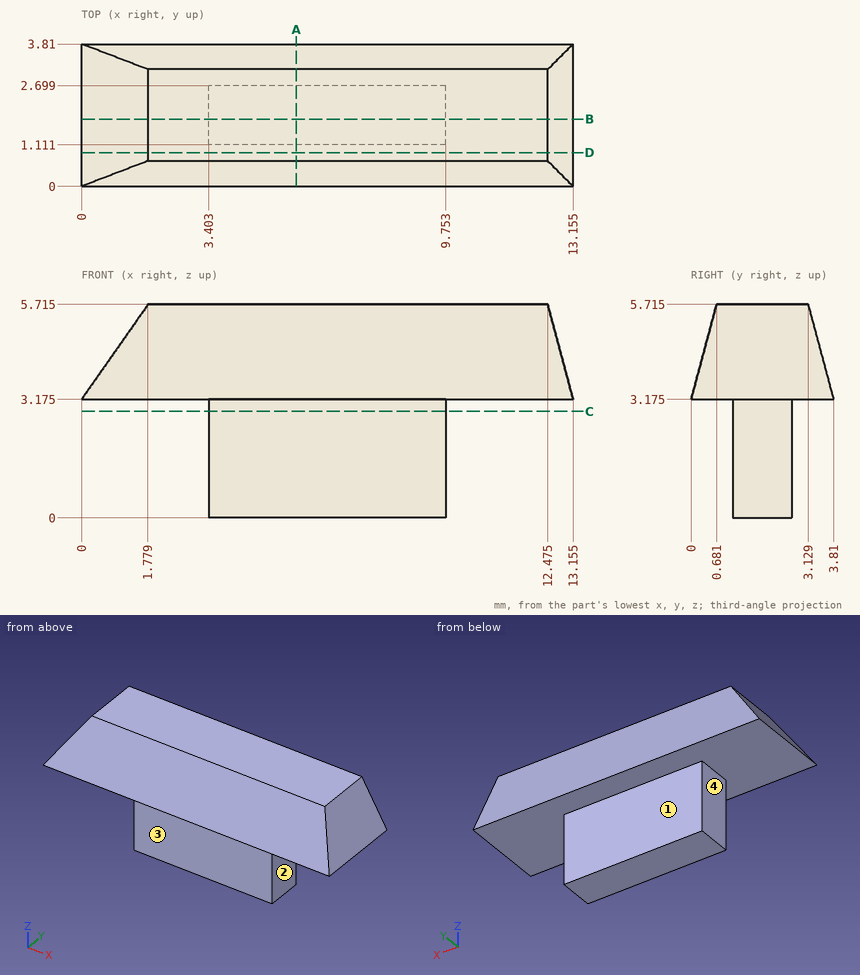
The drawing under review shows one solid part. Ordinate dimensions are in mm from its lowest x, y, z. A direction names the side the tool comes from. Coordinates: 2 decimals unless noted, no trailing zeros. Write each loop counter-clockwise with the first axis right and the second up, starting at its lowest first coordinate (ties: lowest second). Pieces come first, ordered by that corner, then holes. Notation, with made-up numbers: M 42,45 L 52,45 A9 ccw 52,49 Z; hole C -4,75.5 d8. An arc over 180 degrees is marked long. Answer as a JSON object with one key per item and string values.
Item 1: Add section C-C, the plane z = 2.85. Give the boundary of the cut face in (x, y), and give its area (3 significant figures).
Outcome:
{"outline": "M 3.4,1.11 L 9.75,1.11 L 9.75,2.7 L 3.4,2.7 Z", "area": "10.1 mm²"}
Item 2: Add section D-D, the plane y = 0.9. Give the boundary of the cut face in (x, z) (1 decimal), and give its area (3 significant figures).
Outcome:
{"outline": "M 0,3.2 L 13.2,3.2 L 12.5,5.7 L 1.8,5.7 Z", "area": "30.3 mm²"}
Item 3: Insertion check: pin 1 Ø1.5 at (y, z) = (2, 4.5) entering from -X; pin 2 Ø1.7 at (y, z) = (1.5, 1.5) entering from +X; pin 3 Ø1.6 at (x, z) = (7, 2) entering from +Y. Each pin has a flat end and moves straight along its axis. Give the tip position at first contact, or say it passes through.
Outcome:
{"pin 1": "x = 0.4", "pin 2": "x = 9.75", "pin 3": "y = 2.7"}
Item 4: Wall thickness on probe 1 along Z at (x, y) = (11.75, 2.25) (1 decimal); probe 2 along Y at (x, z) = (7.25, 0.45); probe 3 along X at (y, z) = (1.6, 3.5): over which ranges is each line inside the solid? List them lowest first.
Outcome:
{"probe 1": "3.2 to 5.7", "probe 2": "1.11 to 2.7", "probe 3": "0.23 to 13.07"}
Item 5: Machinability: for the marked faces 1, 2, 3 and 4, which of the approach directions +Z, -Z, +X, -X, +Y, -Y give a long, thin tool a straight path to every point of the face, cutting with its end or side? Answer none if there is none.
Outcome:
{"face 1": "-Z, +X, -X, +Y", "face 2": "-Z, +X, +Y, -Y", "face 3": "-Z, +X, -X, -Y", "face 4": "-Z, -X, +Y, -Y"}
Item 6: Add section B-B, the plane y = 1.8. Give the boundary of the cut face in (x, z) (1 decimal).
Outcome:
{"outline": "M 0,3.2 L 3.4,3.2 L 3.4,0 L 9.8,0 L 9.8,3.2 L 13.2,3.2 L 12.5,5.7 L 1.8,5.7 Z"}
Item 7: Add section A-A, the plane x = 5.75. Give the boundary of the cut face in (y, z) (1 decimal), and give its area (3 significant figures).
Outcome:
{"outline": "M 0,3.2 L 1.1,3.2 L 1.1,0 L 2.7,0 L 2.7,3.2 L 3.8,3.2 L 3.1,5.7 L 0.7,5.7 Z", "area": "13.0 mm²"}
